The listing builds one solid part. Answer for the finished solid, in the listing's coordinates (mm). A direction names the side the tool comes from. Round coordinates to 2 decimals unless told otherwise and drop trailing zeros. Loops run counter-clockwise (first coordinate to the right, second up) from the corner with the lowest first, then second, coordinate; pieces in that order, holes last. Notation, with made-up numbers: (35, 38) - (79, 38) arc R25 ccw to (79, 68) - close; hole circle Ø1 at (4.25, 3.5). An arc over 180 degrees is marked (long way). Write item = value, one per line. Start each with the question number.
1) Section B-B, the plane x = 261.5 is taken. Determine the outline of the cut face in (y, z), and give its area (3 significant figures).
2) Section C-C, the plane z = 17.5 is taken. Give the number of separate pieces and of enclosed holes in the cut face, and give its area (3 significant figures).
3) Straight lines are drawn through the part: line 1 along Z through (x, y) = (239, 70); line 2 along Y through (x, z) = (304, -14); line 3 along Y through (x, z) = (220, 13.75). For each, find the intervals that lie inside material, in ascending order.
4) Given pin 1 Ø7.5 at (x, z) = (319, -16) entering from +Y; pin 2 Ø1 at (y, z) = (52, 2.5) entering from -X; pin 3 Ø3 at (y, z) = (34, -13.5) entering from +X, each flat-ended and moving along its own axis, determine where each tip first touches the part or whether it passes through.
5) Section D-D, the plane y = 57.5 is taken. Determine the outline of the cut face in (x, z).
6) For a pull along X with two mould halves and no side action, classify faces 4 (the flat face through (361.133, 32.254, 0.294)), 5 (the flat face through (318.5, 27.53, 0.29)), 6 (the flat face through (282, 25, 0)) as released by +X, released by -X, zero draft, split by the parting line, or undercut.
7) A tool of negligible diameter and unlimited length cuts with its end or side. For faces 1 (the flat face through (222, 38, -11)), 2 (the cylindrical face through (225.97, 66.39, -0.29)), 3 (the flat face through (242.67, 54.47, 13.6)), from which of +Z, -Z, +X, -X, +Y, -Y can it reach the whole face along a straight path? Write none if from no direction.
from build123d import *

# Parameters (mm, degrees)
SKETCH_1_R             = 2.5
EXTRUDE_1_DEPTH        = 21
CUT_EXTRUDE_1_DEPTH    = 11
CUT_EXTRUDE_2_DEPTH    = 15
CUT_EXTRUDE_3_DEPTH    = 25
PATTERN_LINEAR_1_COUNT = 8
PATTERN_LINEAR_1_PITCH = 10


with BuildPart() as part:
    # 草图1 → 凸台-拉伸1 (new, symmetric)
    with BuildSketch(Plane.XY):
        with BuildLine():
            Line((218.502541787, 68.048442919), (210.340741737, 37.588190451))
            ThreePointArc((210.340741737, 37.588190451), (212.066466597, 28.91238571), (220, 25))
            Line((220, 25), (358.547941324, 25))
            Line((358.547941324, 25), (370, 25))
            Line((370, 25), (346.78040334, 43.996060933))
            Line((346.78040334, 43.996060933), (230.908606215, 75.200654039))
            ThreePointArc((230.908606215, 75.200654039), (223.222977943, 74.196224157), (218.502541787, 68.048442919))
        make_face()
        with Locations(Location((220, 35, 0), (0, 0, 180))):
            Circle(SKETCH_1_R, mode=Mode.SUBTRACT)
        with Locations(Location((228.27716468, 65.429340608, 0), (0, 0, 180))):
            Circle(SKETCH_1_R, mode=Mode.SUBTRACT)
    extrude(amount=EXTRUDE_1_DEPTH, both=True)

    # 草图2 → 切除-拉伸1 (cut, symmetric)
    with BuildSketch(Plane.XY):
        with BuildLine():
            Line((235, 20), (235, 35))
            ThreePointArc((235, 35), (230.606601718, 45.606601718), (220, 50))
            Line((220, 50), (205, 50))
            Line((205, 50), (205.078251443, 33.469830071))
            Line((205.078251443, 33.469830071), (205.078251443, 20))
            Line((205.078251443, 20), (235, 20))
        make_face()
    extrude(amount=CUT_EXTRUDE_1_DEPTH, both=True, mode=Mode.SUBTRACT)

    # 草图3 → 切除-拉伸2 (cut)
    with BuildSketch(Plane.XY.offset(21)):
        Polygon((237.599806566, 73.398695413), (247.888705992, 35), (366.823980308, 35), (338.386105999, 70.333701244), align=None)
    cut_extrude_2 = extrude(amount=-CUT_EXTRUDE_2_DEPTH, mode=Mode.SUBTRACT)

    # 镜向1: 切除-拉伸2 across plane
    add(cut_extrude_2.mirror(Plane.XY), mode=Mode.SUBTRACT)

    # 草图4 → 切除-拉伸3 (cut, symmetric)
    with BuildSketch(Plane.XY):
        Polygon((262.071941238, 21.339745962), (267.071941238, 30), (272.071941238, 21.339745962), align=None)
    cut_extrude_3 = extrude(amount=CUT_EXTRUDE_3_DEPTH, both=True, mode=Mode.SUBTRACT)

    # 阵列(线性)1: 切除-拉伸3 ×8
    with Locations(*[(i * PATTERN_LINEAR_1_PITCH, 0, 0) for i in range(1, PATTERN_LINEAR_1_COUNT)]):
        add(cut_extrude_3, mode=Mode.SUBTRACT)


solid = part.part
Geometry check:
q1.outline = (25, -21) - (35, -21) - (35, -6) - (66.96, -6) - (66.96, 6) - (35, 6) - (35, 21) - (25, 21) - close
q1.area = 804 mm2
q2.separate_pieces = 1
q2.enclosed_holes = 2
q2.area = 2,450 mm2
q3.line_1 = -6 to 6
q3.line_2 = 25 to 35
q3.line_3 = 25 to 32.5, 37.5 to 71.25
q4.pin_1 = 35
q4.pin_2 = 214.07
q4.pin_3 = 360.83
q5.outline = (215.68, -21) - (241.86, -21) - (241.86, -6) - (296.64, -6) - (296.64, 6) - (241.86, 6) - (241.86, 21) - (215.68, 21) - close
q6.face_4 = released by +X
q6.face_5 = undercut
q6.face_6 = zero draft
q7.face_1 = -X, -Y
q7.face_2 = +Z, -Z
q7.face_3 = +Z, +X, +Y
